```python
from build123d import *

# Parameters (mm, degrees)
F0_W        = 6
F0_H        = 20.5
F0_H_2      = 4
F0_H_3      = 6
F1_DEPTH    = 15
F2_T1_DEPTH = 15
F2_T3_DEPTH = 16.4497757802
F2_T5_DEPTH = 16.6588870729
F2_T7_DEPTH = 18.75
F3_R        = 2.075
F4_DEPTH    = 12.5


# Not quite as in the source:
# - a fillet or chamfer that OpenCascade refuses, or shapes differently, is made with other operations: its cross-section is extruded or revolved along the edge and cut away or added


with BuildPart() as f1:
    # F0 (on Front) → F1 (new body)
    with BuildSketch(Plane.XZ):
        Polygon((-3, 2.3), (-3, 0), (3, 0), (3, 2.3), (7, 2.3), (7, 3.3), (3, 7.7), (-3, 7.7), (-7, 3.3), (-7, 2.3), align=None)
        with Locations((0, -10.25)):
            Rectangle(F0_W, F0_H)
        with Locations((0, -22.5)):
            Rectangle(F0_W, F0_H_2)
        with Locations((0, -27.5)):
            Rectangle(F0_W, F0_H_3)
    extrude(amount=F1_DEPTH)

    # F2: fillet of radius 0.75 on 10 edges, made by hand

    # F2_s2 → F2_t1 (join)
    with BuildSketch(Plane.XZ):
        with BuildLine():
            ThreePointArc((-3, 1.55), (-3.2196699141, 2.0803300859), (-3.75, 2.3))
            Line((-3.75, 2.3), (-3, 2.3))
            Line((-3, 2.3), (-3, 1.55))
        make_face()
        with BuildLine():
            ThreePointArc((3, 1.55), (3.2196699141, 2.0803300859), (3.75, 2.3))
            Line((3.75, 2.3), (3, 2.3))
            Line((3, 2.3), (3, 1.55))
        make_face()
    extrude(amount=F2_T1_DEPTH)

    # F2_s4 → F2_t3 (cut)
    with BuildSketch(Plane.XZ.offset(-0.7248878901)):
        with BuildLine():
            ThreePointArc((7, 3.010044844), (6.9495413824, 3.2804923515), (6.804955055, 3.5145494394))
            Line((6.804955055, 3.5145494394), (7, 3.3))
            Line((7, 3.3), (7, 3.010044844))
        make_face()
        with BuildLine():
            ThreePointArc((-6.804955055, 3.5145494394), (-6.9495413824, 3.2804923515), (-7, 3.010044844))
            Line((-7, 3.010044844), (-7, 3.3))
            Line((-7, 3.3), (-6.804955055, 3.5145494394))
        make_face()
    extrude(amount=F2_T3_DEPTH, mode=Mode.SUBTRACT)

    # F2_s6 → F2_t5 (cut)
    with BuildSketch(Plane.XZ.offset(-0.8294435365)):
        with BuildLine():
            ThreePointArc((3.2231776405, 7.4545045955), (2.971637774, 7.6358857218), (2.6682225854, 7.7))
            Line((2.6682225854, 7.7), (3, 7.7))
            Line((3, 7.7), (3.2231776405, 7.4545045955))
        make_face()
        with BuildLine():
            ThreePointArc((-2.6682225854, 7.7), (-2.971637774, 7.6358857218), (-3.2231776405, 7.4545045955))
            Line((-3.2231776405, 7.4545045955), (-3, 7.7))
            Line((-3, 7.7), (-2.6682225854, 7.7))
        make_face()
    extrude(amount=F2_T5_DEPTH, mode=Mode.SUBTRACT)

    # F2_s8 → F2_t7 (cut)
    with BuildSketch(Plane.XZ.offset(-1.875)):
        with BuildLine():
            ThreePointArc((-7, 3.05), (-6.7803300859, 2.5196699141), (-6.25, 2.3))
            Line((-6.25, 2.3), (-7, 2.3))
            Line((-7, 2.3), (-7, 3.05))
        make_face()
        with BuildLine():
            ThreePointArc((6.25, 2.3), (6.7803300859, 2.5196699141), (7, 3.05))
            Line((7, 3.05), (7, 2.3))
            Line((7, 2.3), (6.25, 2.3))
        make_face()
        with BuildLine():
            ThreePointArc((2.25, -30.5), (2.7803300859, -30.2803300859), (3, -29.75))
            Line((3, -29.75), (3, -30.5))
            Line((3, -30.5), (2.25, -30.5))
        make_face()
        with BuildLine():
            ThreePointArc((-3, -29.75), (-2.7803300859, -30.2803300859), (-2.25, -30.5))
            Line((-2.25, -30.5), (-3, -30.5))
            Line((-3, -30.5), (-3, -29.75))
        make_face()
    extrude(amount=F2_T7_DEPTH, mode=Mode.SUBTRACT)

    # F3 (on Right) → F4 (cut, symmetric)
    with BuildSketch(Plane.YZ):
        with Locations((-7.5, -22.575)):
            Circle(F3_R)
    extrude(amount=F4_DEPTH, both=True, mode=Mode.SUBTRACT)


solid = f1.part
```
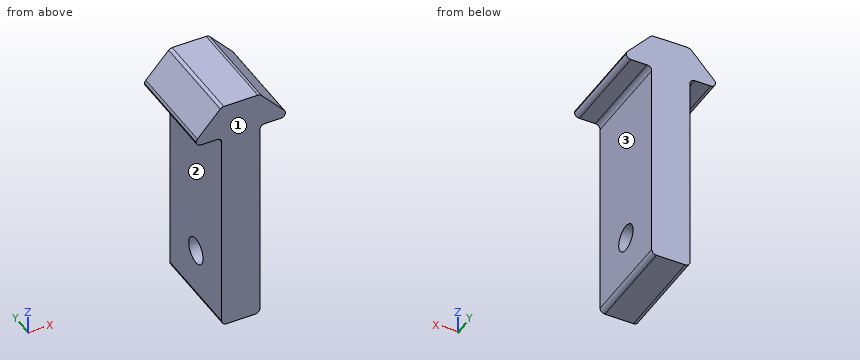
For this review, take the finished solid that the model builds, in its own axes (mm). Face numbers are marked on the shaded views. A direction names the side the tool comes from. Coordinates: 2 decimals unless noted, no trailing zeros. Order: outer loops, then holes, each group sorted by start corner. A loop starts at its lowest first (then second) coordinate and runs counter-clockwise, first axis right, second up. Notation, with made-up numbers: (30, 11.25) -> (83, 11.25) arc R23 cw to (83, 40.25) -> close; hole circle Ø10 at (50.25, 73.5). An arc over 180 degrees is marked (long way). Use CSV: the item, a comma, the result in double quotes. Start each with the question number.
Item 1: Insertion check: pin 1 (2 mm diameter, centred on y = -3, z = -9.5, fed in from -X); pin 2 (3 mm diameter, centred on x = -5.5, y = -11, fed in from -Z); pin 3 (2 mm diameter, centred on y = -11, z = 0.5, fed in from +X). Each pin has a flat end and moves straight along its axis. Give the tip position at first contact, or say it passes through.
Item 2: We need section C-C, the plane z = -14. Give the boundary of the cut face in (x, y), then the cut area to 3 significant figures.
Item 3: We need section B-B, the plane y = -13.5. Give the boundary of the cut face in (x, z).
Item 4: We need section A-A, the plane y = -7.5. Give the boundary of the cut face in (x, z).
Item 5: For the marked faces 1, 2 and 3, list the 3-axis set-ups (+Z, -Z, +X, -X, +Y, -Y) from which the entire face can be reached by the end or side of a thin tool; tool diameter is ignored.
Item 6: Wall thickness on probe 1 along Z at (x, y) = (-0.4, -7.5); probe 2 along X at (y, z) = (-10.25, -23.5); probe 3 along Z at (x, y) = (-2, -8.75): over which ranges is each line inside the solid? List them lowest first.
Derived:
1,pin 1,"stops at x = -3"
1,pin 2,"stops at z = 2.3"
1,pin 3,"stops at x = 3"
2,outline,"(-3, -15) -> (3, -15) -> (3, 0) -> (-3, 0) -> close"
2,area,"90.0 mm^2"
3,outline,"(-7, 3.03) arc R0.75 ccw to (-6.25, 2.3) -> (-3.75, 2.3) arc R0.75 cw to (-3, 1.55) -> (-3, -29.75) arc R0.75 ccw to (-2.25, -30.5) -> (2.25, -30.5) arc R0.75 ccw to (3, -29.75) -> (3, 1.55) arc R0.75 cw to (3.75, 2.3) -> (6.25, 2.3) arc R0.75 ccw to (7, 3.03) arc R0.75 ccw to (6.8, 3.51) -> (3.22, 7.45) arc R0.75 ccw to (2.67, 7.7) -> (-2.67, 7.7) arc R0.75 ccw to (-3.22, 7.45) -> (-6.8, 3.51) arc R0.75 ccw to start"
4,outline,"(-7, 3.03) arc R0.75 ccw to (-6.25, 2.3) -> (-3.75, 2.3) arc R0.75 cw to (-3, 1.55) -> (-3, -20.5) -> (3, -20.5) -> (3, 1.55) arc R0.75 cw to (3.75, 2.3) -> (6.25, 2.3) arc R0.75 ccw to (7, 3.03) arc R0.75 ccw to (6.8, 3.51) -> (3.22, 7.45) arc R0.75 ccw to (2.67, 7.7) -> (-2.67, 7.7) arc R0.75 ccw to (-3.22, 7.45) -> (-6.8, 3.51) arc R0.75 ccw to start; (-3, -29.75) arc R0.75 ccw to (-2.25, -30.5) -> (2.25, -30.5) arc R0.75 ccw to (3, -29.75) -> (3, -24.65) -> (-3, -24.65) -> close"
5,face 1,"+Z, -Z, +X, -X, -Y"
5,face 2,"-Z, -X, +Y, -Y"
5,face 3,"-Z, +X, +Y, -Y"
6,probe 1,"z = -30.5 to -24.65, -20.5 to 7.7"
6,probe 2,"x = -3 to 3"
6,probe 3,"z = -30.5 to -24.23, -20.92 to 7.7"
